Can you work these out from the model? Positions are in its coordinate system, mm. Face numbers are marked on the shaded views. A direction names the side the tool comes from. Round coordinates to 2 decimals unless told otherwise and drop trailing zeros. Loops run counter-clockwise (first coordinate to the right, second up) from the corner with the lowest first, then second, coordinate; pieces in that order, holes last. Notation, with made-up numbers: M 40.5,24.25 L 44.5,24.25 A18 ccw 44.5,45.25 Z; hole C 81.25,-30.5 d3. An arc over 180 degrees is marked long. Return JSON: item names as keys, results as strings.
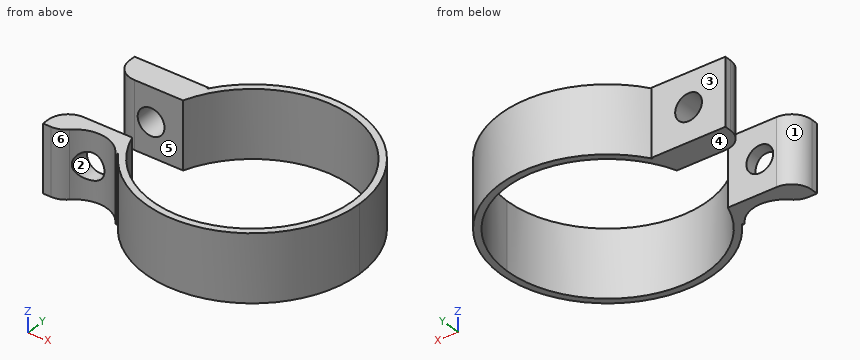
```python
from build123d import *

# Parameters (mm, degrees)
SALIENTE_EXTRUIR4_DEPTH = 10
REDONDEO4_R             = 3
CROQUIS4_R              = 2
CORTAR_EXTRUIR1_DEPTH   = 21
CROQUIS5_R              = 4.836264875
CORTAR_EXTRUIR2_DEPTH   = 21
REDONDEO5_R             = 3


with BuildPart() as part:
    # Croquis1 → Saliente-Extruir4 (new body)
    with BuildSketch(Plane.XY):
        with BuildLine():
            ThreePointArc((-15.198684154, 5), (-14.424283954, 6.923874089), (-13.407545238, 8.731422032))
            Line((-13.407545238, 8.731422032), (-13.407545238, 9))
            Line((-13.407545238, 9), (-24.407545238, 9))
            Line((-24.407545238, 9), (-24.407545238, 5))
            Line((-24.407545238, 5), (-15.198684154, 5))
        make_face()
        with BuildLine():
            Line((15, 0), (16, 0))
            ThreePointArc((16, 0), (4.554079281, 15.338199435), (-13.407545238, 8.731422032))
            ThreePointArc((-13.407545238, 8.731422032), (-14.424283954, 6.923874089), (-15.198684154, 5))
            Line((-15.198684154, 5), (-14.142135624, 5))
            ThreePointArc((-14.142135624, 5), (2.536529681, 14.783978395), (15, 0))
        make_face()
        with BuildLine():
            Line((-13.407545238, -9), (-13.407545238, -8.731422032))
            ThreePointArc((-13.407545238, -8.731422032), (-14.424283954, -6.923874089), (-15.198684154, -5))
            Line((-15.198684154, -5), (-24.407545238, -5))
            Line((-24.407545238, -5), (-24.407545238, -9))
            Line((-24.407545238, -9), (-13.407545238, -9))
        make_face()
        with BuildLine():
            ThreePointArc((-13.407545238, -8.731422032), (4.554079281, -15.338199435), (16, 0))
            Line((16, 0), (15, 0))
            ThreePointArc((15, 0), (2.536529681, -14.783978395), (-14.142135624, -5))
            Line((-14.142135624, -5), (-15.198684154, -5))
            ThreePointArc((-15.198684154, -5), (-14.424283954, -6.923874089), (-13.407545238, -8.731422032))
        make_face()
    extrude(amount=SALIENTE_EXTRUIR4_DEPTH)

    # Redondeo4
    redondeo4_edges = [part.edges().sort_by_distance(p)[0] for p in [
        (-24.407545238, 5, 5),
        (-24.407545238, -5, 5),
    ]]
    fillet(redondeo4_edges, radius=REDONDEO4_R)

    # Croquis4 → Cortar-Extruir1 (cut)
    with BuildSketch(Plane(origin=(0, 9, 0), x_dir=(1, 0, 0), z_dir=(0, 1, 0))):
        with Locations((-18.907545238, -5)):
            Circle(CROQUIS4_R)
    extrude(amount=-CORTAR_EXTRUIR1_DEPTH, mode=Mode.SUBTRACT)

    # Croquis5 → Cortar-Extruir2 (cut)
    with BuildSketch(Plane(origin=(0, 0, 0), x_dir=(-1, 0, 0), z_dir=(0, 0, -1))):
        with Locations((17.698992991, -11.582378958)):
            Circle(CROQUIS5_R)
    extrude(amount=-CORTAR_EXTRUIR2_DEPTH, mode=Mode.SUBTRACT)

    # Redondeo5
    redondeo5_edges = [part.edges().sort_by_distance(p)[0] for p in [
        (-21.788097643, -9, 5),
    ]]
    fillet(redondeo5_edges, radius=REDONDEO5_R)


solid = part.part
```
Q1. Suppose I cut it at A-A, the plane z = 5.5. Please give me the cut outline in (x, y), plus the area to 3 significant figures.
Results:
{"outline": "M -24.41,-9 L -23.2,-9 A3 ccw -21.09,-8.14 A4.84 cw -20.84,-7.91 L -20.84,-5 L -21.41,-5 A3 ccw -24.41,-8 Z; M -24.41,8 A3 ccw -21.41,5 L -20.84,5 L -20.84,9 L -24.41,9 Z; M -16.97,-6.8 A4.84 cw -13.61,-9 L -13.41,-9 L -13.41,-8.73 A16 ccw long -13.41,8.73 L -13.41,9 L -16.97,9 L -16.97,5 L -14.14,5 A15 cw long -14.14,-5 L -16.97,-5 Z", "area": "127 mm2"}
Q2. If I drill on line 1 along Y through (x, z) = (0, 4); line 2 along X through (y, z) = (6.3, 5); line 3 along X through (y, z) = (7.65, 5), over which ranges is the centre line in solid material (lowest first)?
Results:
{"line 1": "y = -16 to -15, 15 to 16", "line 2": "x = -23.88 to -20.91, -16.91 to -13.61, 13.61 to 14.71", "line 3": "x = -24.39 to -20.91, -16.91 to -12.9, 12.9 to 14.05"}
Q3. Suppose I cut it at C-C, the plane z = 9. Please give me the cut outline in (x, y), plus the area to 3 significant figures.
Results:
{"outline": "M -24.41,-9 L -23.2,-9 A3 ccw -21.09,-8.14 A4.84 cw -13.61,-9 L -13.41,-9 L -13.41,-8.73 A16 ccw long -13.41,8.73 L -13.41,9 L -24.41,9 L -24.41,8 A3 ccw -21.41,5 L -14.14,5 A15 cw long -14.14,-5 L -21.41,-5 A3 ccw -24.41,-8 Z", "area": "151 mm2"}
Q4. Thinking about a two-plate mould opening in X: for the marked faces 1, 2 and 3, which applies, pulls with the +X half, pulls with the -X half, needs draft (parallel to the pull), parting line crosses it, or undercut?
Results:
{"face 1": "pulls with the -X half", "face 2": "undercut", "face 3": "needs draft"}
Q5. Suppose I cut it at B-B, the plane x = 3. Please give me the cut outline in (y, z).
Results:
{"outline": "M -15.72,0 L -14.7,0 L -14.7,10 L -15.72,10 Z; M 14.7,0 L 15.72,0 L 15.72,10 L 14.7,10 Z"}
Q6. I'm going to push flat-ended pins straight in: pin 1 Ø1.3 at (x, z) = (-23.5, 4) entering from -Y; pin 2 Ø3 at (x, z) = (-16, 6.5) entering from +Y; pin 3 Ø5 at (x, z) = (-18.91, 5) entering from -Y; pin 4 Ø10 at (x, y) = (-3, -5.5) entering from +Z. Where does each tip first touch, or does it pass through?
Results:
{"pin 1": "stops at y = -9", "pin 2": "stops at y = 9", "pin 3": "stops at y = -8.41", "pin 4": "passes through"}
Q7. On a 3-axis mill with a long thin cutter (end or side, diameter ignored), from which of +Z, -Z, +X, -X, +Y, -Y can I reach the whole of each face in a straight line? I mean the marked faces 4, 5 and 6. Say none if no direction works.
Results:
{"face 4": "-Z, +X, -X, +Y, -Y", "face 5": "+Z, -Z, -X", "face 6": "+Z, -Z, -Y"}
Q8. Suppose I cut it at D-D, the plane y = -13. Please give me the cut outline in (x, z), plus the area to 3 significant figures.
Results:
{"outline": "M -9.33,0 L -7.48,0 L -7.48,10 L -9.33,10 Z; M 7.48,0 L 9.33,0 L 9.33,10 L 7.48,10 Z", "area": "36.9 mm2"}
